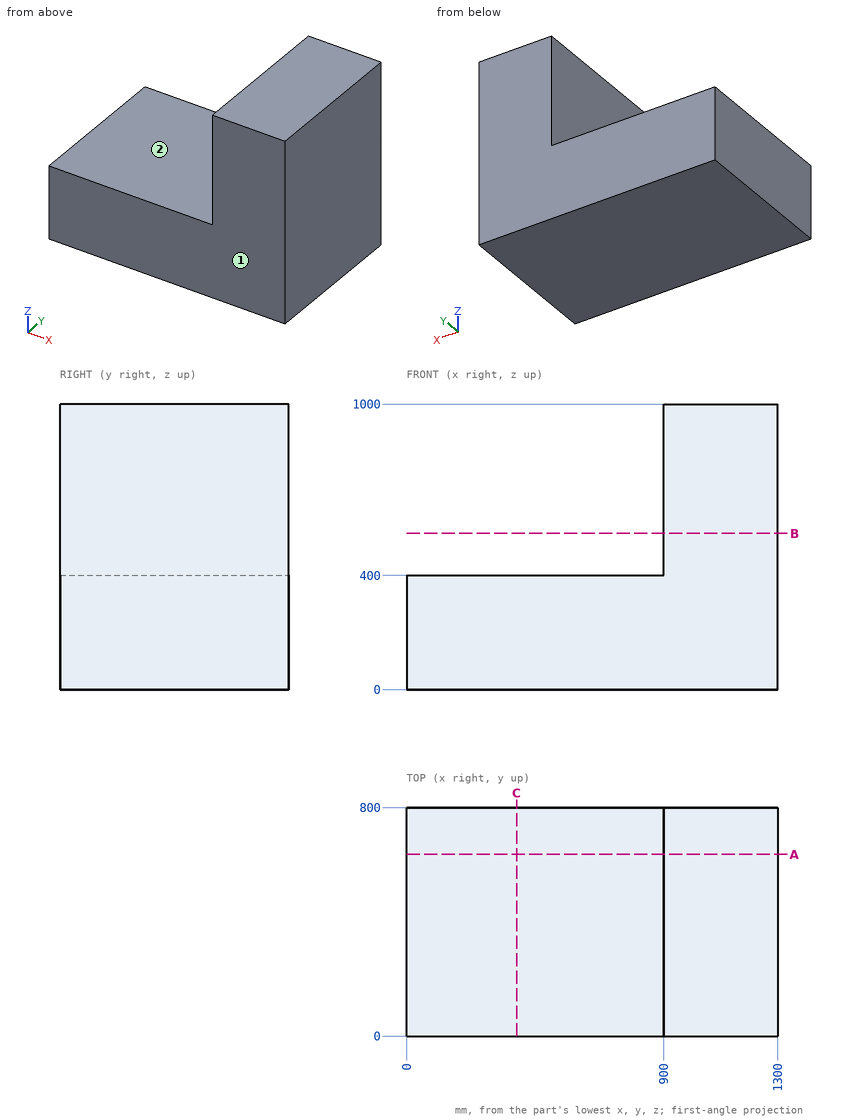
Design review of the part shown in the three views and the two pictorial views. Dimensions are in mm from the part's minimum x, y and z. A direction names the side the tool comes from. Round coordinates to 2 decimals unless told otherwise and drop trailing zeros. Order: outer loops, then holes, each group sorted by start corner. A loop starts at its lowest first (then second) coordinate and runs counter-clockwise, first axis right, second up. Notation, with made-up numbers: M -21.75,50 L 29.25,50 A19 cw 29.25,65 Z; hole C 3,-17.75 d10. An arc over 180 degrees is marked long. Put each result on its own line as item: value.
Q1. Consider section C-C (x = 385). State the section outline as (y, z) points, and give its area (3 significant figures).
Reported:
outline: M 0,0 L 800,0 L 800,400 L 0,400 Z
area: 320,000 mm²
Q2. Consider section B-B (z = 547). State the section outline as (x, y) points, and give its area (3 significant figures).
Reported:
outline: M 900,0 L 1300,0 L 1300,800 L 900,800 Z
area: 320,000 mm²
Q3. To check wall thickness, follow line 1 (X direction, y = 426.5, z = 935.5); line 2 (Z direction, x = 502, y = 493.5). State the ranges of each line that lie inside material, in increasing order.
Reported:
line 1: 900 to 1300
line 2: 0 to 400
Q4. Machinability: for the marked faces 1 and 2, which of the approach directions +Z, -Z, +X, -X, +Y, -Y give a long, thin tool a straight path to every point of the face, cutting with its end or side? Answer none if there is none.
Reported:
face 1: +Z, -Z, +X, -X, -Y
face 2: +Z, -X, +Y, -Y
Q5. Insertion check: pin 1 Ø12 at (x, y) = (1006.5, 163) entering from -Z; pin 2 Ø4 at (x, y) = (485, 679.5) entering from +Z; pin 3 Ø12 at (y, z) = (628, 794.5) entering from -X. Each pin has a flat end and moves straight along its axis. Give the tip position at first contact, or say it passes through.
Reported:
pin 1: z = 0
pin 2: z = 400
pin 3: x = 900
Q6. Consider section A-A (y = 636). State the section outline as (x, z) points.
Reported:
outline: M 0,0 L 1300,0 L 1300,1000 L 900,1000 L 900,400 L 0,400 Z
